Work out the finished part from the listing and answer in its coordinate system (mm). A direction names the side the tool comes from. Round coordinates to 2 decimals unless told otherwise and drop trailing zeros. Order: outer loops, then holes, each group sorted by start corner. A loop starts at its lowest first (then second) coordinate and runs counter-clockwise, first axis right, second up. Notation, with made-up numbers: (53, -38) - (69, -38) arc R17 ccw to (69, -17) - close; hole circle Ø2 at (-37, -8.75). An arc over 180 degrees is marked (long way). Put each result on its own line as item: value.
```python
from build123d import *

# Parameters (mm, degrees)
F0_R         = 4
F1_DEPTH     = 15
F3_W         = 15
F3_H         = 15
F3_R         = 2
F4_DEPTH     = 7
F6_W         = 15
F6_H         = 15
F6_R         = 2
F7_DEPTH     = 7
F8_W         = 5.4
F8_H         = 15
F8_R         = 1.5
F9_DEPTH     = 5
F10_DEPTH    = 20
F12_W        = 5.4
F12_H        = 2.5
F12_W_2      = 7.6
F12_H_2      = 15
F12_R        = 1.5
F13_DEPTH    = 5
F12_W_3      = 2.2
F12_H_3      = 2
F14_DEPTH    = 3
F15_T4_DEPTH = 27.2150489639
F16_SIZE     = 2


# Not quite as in the source:
# - a fillet or chamfer that OpenCascade refuses, or shapes differently, is made with other operations: its cross-section is extruded or revolved along the edge and cut away or added


with BuildPart() as f1:
    # F0 (on Top) → F1 (new body)
    with BuildSketch(Plane.XY):
        Polygon((12.5, -12.5), (12.5, 12.5), (-12.5, 12.5), (-12.5, -12.5), (-5.5, -12.5), (-5.5, -7), (5.5, -7), (5.5, -12.5), align=None)
        Circle(F0_R, mode=Mode.SUBTRACT)
    extrude(amount=F1_DEPTH)

    # F3 (on offset) → F4 (join)
    with BuildSketch(Plane(origin=(-12.5, 0, 0), x_dir=(0, -1, 0), z_dir=(-1, 0, 0))):
        with Locations((20, 7.5)):
            Rectangle(F3_W, F3_H)
        with Locations((20, 7.5)):
            Circle(F3_R, mode=Mode.SUBTRACT)
    extrude(amount=-F4_DEPTH)

    # F6 (on offset) → F7 (join)
    with BuildSketch(Plane.YZ.offset(12.5)):
        with Locations((-20, 7.5)):
            Rectangle(F6_W, F6_H)
        with Locations((-20, 7.5)):
            Circle(F6_R, mode=Mode.SUBTRACT)
    extrude(amount=-F7_DEPTH)

    # F8 (on offset) → F9 (join)
    with BuildSketch(Plane(origin=(-12.5, 0, 0), x_dir=(0, -1, 0), z_dir=(-1, 0, 0))):
        with Locations((-15.2, 7.5)):
            Rectangle(F8_W, F8_H)
        with Locations((-14.4, 2.5)):
            Circle(F8_R, mode=Mode.SUBTRACT)
        with Locations((-14.4, 12.5)):
            Circle(F8_R, mode=Mode.SUBTRACT)
    extrude(amount=-F9_DEPTH)

    # F8 (on offset) → F10 (join)
    with BuildSketch(Plane(origin=(-12.5, 0, 0), x_dir=(0, -1, 0), z_dir=(-1, 0, 0))):
        with Locations((-15.2, 7.5)):
            Rectangle(F8_W, F8_H)
        with Locations((-14.4, 2.5)):
            Circle(F8_R, mode=Mode.SUBTRACT)
        with Locations((-14.4, 12.5)):
            Circle(F8_R, mode=Mode.SUBTRACT)
    extrude(amount=F10_DEPTH)

    # F12 (on offset) → F13 (join)
    with BuildSketch(Plane(origin=(-32.5, 0, 0), x_dir=(0, -1, 0), z_dir=(-1, 0, 0))):
        with Locations((-15.2, 16.25)):
            Rectangle(F12_W, F12_H)
        Polygon((30, 19.5), (30, 17.5), (37.6, 17.5), (37.6, 24.5), (-17.9, 24.5), (-17.9, 17.5), (-12.5, 17.5), (-12.5, 19.5), (-10.3, 19.5), align=None)
        with Locations((33.8, 16.25)):
            Rectangle(F12_W_2, F12_H)
        with Locations((33.8, 7.5)):
            Rectangle(F12_W_2, F12_H_2)
        with Locations((34.1, 2.5)):
            Circle(F12_R, mode=Mode.SUBTRACT)
        with Locations((34.1, 12.5)):
            Circle(F12_R, mode=Mode.SUBTRACT)
    extrude(amount=-F13_DEPTH)

    # F12 (on offset) → F14 (join)
    with BuildSketch(Plane(origin=(-32.5, 0, 0), x_dir=(0, -1, 0), z_dir=(-1, 0, 0))):
        with Locations((-11.4, 7.5)):
            Rectangle(F12_W_3, F12_H_2)
        with Locations((-11.4, 16.25)):
            Rectangle(F12_W_3, F12_H)
        with Locations((-11.4, 18.5)):
            Rectangle(F12_W_3, F12_H_3)
    extrude(amount=-F14_DEPTH)

    # F15: chamfer of 3 on 1 edges, made by hand


with BuildPart() as f15_tool2:
    # F15_s3 → F15_t4 (new body)
    with BuildSketch(Plane.XY.offset(-7.7150489639)):
        Polygon((-29.5, 13.3), (-32.5, 10.3), (-29.5, 10.3), align=None)
    extrude(amount=F15_T4_DEPTH)

    split(bisect_by=Plane.XZ.offset(-12.5), keep=Keep.TOP)


with BuildPart() as f1_1:
    add(f1.part)

    # F15_t1: cut F15_tool2
    add(f15_tool2.part, mode=Mode.SUBTRACT)

    # F16
    f16_edges = [f1_1.edges().sort_by_distance(p)[0] for p in [
        (-27.5, -30, 9.75),
    ]]
    chamfer(f16_edges, length=F16_SIZE)


solid = f1_1.part
```
1) For a pull along X with two mould halves and no side action, classify faces 1 (the cylindrical face through (-0.867, -3.905, 7.395)), 2 (the flat face through (-7.5, 15, 8)), 3 (the flat face through (-23, 17.9, 10)) as pulls with the +X half, pulls with the -X half, needs draft (parallel to the pull), parting line crosses it, or undercut.
Findings below:
face 1: undercut
face 2: pulls with the +X half
face 3: needs draft
2) A cutting plane is placed at C-C on y = 0. Write down the section's boundary in (x, z).
Findings below:
outline: (-32.5, 19.5) - (-27.5, 19.5) - (-27.5, 24.5) - (-32.5, 24.5) - close; (-12.5, 0) - (-4, 0) - (-4, 15) - (-12.5, 15) - close; (4, 0) - (12.5, 0) - (12.5, 15) - (4, 15) - close
3) A cutting plane is placed at B-B on x = 0. Write down the section's boundary in (y, z), then the cut area to 4 significant figures.
Findings below:
outline: (-7, 0) - (-4, 0) - (-4, 15) - (-7, 15) - close; (4, 0) - (12.5, 0) - (12.5, 15) - (4, 15) - close
area: 172.5 mm2
4) Straight lines are drawn through the part: L1, parallel to Z at x = -13.5, y = 14.4; L2, parallel to Z at x = -28.95, y = -34.1; L3, parallel to Y at x = 0, z = 4.75. For each, find the intervals that lie inside material, in ascending order. Write a range as from..to.
Findings below:
L1: z = 0..1, 4..11, 14..15
L2: z = 0..1, 4..11, 14..24.5
L3: y = -7..-4, 4..12.5
5) For faces 4 (the flat face through (-28.5, -31, 9.9)), 5 (the flat face through (3, 12.5, 7)), 6 (the flat face through (-30, -10, 24.5)), 7 (the flat face through (-5.5, -17, 8)), 8 (the cylindrical face through (-9.049, -18.526, 8.852)), determine the directions among +Z, -Z, +X, -X, +Y, -Y from which every point of the face is accessible in a straight line to the end or side of a thin tool.
Findings below:
face 4: -Z, +X
face 5: +Z, -Z, +X, +Y
face 6: +Z, +X, -X, +Y, -Y
face 7: +Z, -Z, -Y
face 8: +X, -X
6) Given pin 1 Ø1.5 at (x, y) = (-30, -14) entering from -Z; pin 2 Ø2 at (x, y) = (-11, -26) entering from -Z; pin 3 Ø5.5 at (x, z) = (-20.5, 12) entering from -Y; pin 4 Ø5.5 at (x, z) = (-2.5, 11) entering from -Y, each flat-ended and moving along its own axis, determine where each tip first touches the part or whether it passes through.
Findings below:
pin 1: stops at z = 19.5
pin 2: stops at z = 0
pin 3: stops at y = 12.5
pin 4: stops at y = -7
7) A cutting plane is placed at D-D on z = 17. Write down the section's boundary in (x, y), then the cut area to 3 significant figures.
Findings below:
outline: (-32.5, -37.6) - (-27.5, -37.6) - (-27.5, -32) - (-29.5, -30) - (-32.5, -30) - close; (-32.5, 10.3) - (-30.3, 12.5) - (-27.5, 12.5) - (-27.5, 17.9) - (-32.5, 17.9) - close
area: 65.4 mm2
8) A cutting plane is placed at A-A on z = 7.5. Write down the section's boundary in (x, y), then the cut area to 3 significant figures.
Findings below:
outline: (-32.5, -37.6) - (-27.5, -37.6) - (-27.5, -32) - (-29.5, -30) - (-32.5, -30) - close; (-32.5, 10.3) - (-30.3, 12.5) - (-12.5, 12.5) - (-12.5, -18) - (-5.5, -18) - (-5.5, -7) - (5.5, -7) - (5.5, -18) - (12.5, -18) - (12.5, 12.5) - (-7.5, 12.5) - (-7.5, 17.9) - (-32.5, 17.9) - close; (-12.5, -27.5) - (-5.5, -27.5) - (-5.5, -22) - (-12.5, -22) - close; (5.5, -27.5) - (12.5, -27.5) - (12.5, -22) - (5.5, -22) - close; hole circle Ø8 at (0, 0)
area: 842 mm2
